from build123d import *

# Parameters (mm, degrees)
SKETCH_1_R               = 8
EXTRUDE_1_DEPTH          = 32
M6X1_0_1_D               = 5
M6X1_0_1_DEPTH           = 6
M6X1_0_1_TIP             = 1.502151548
M6X1_0_2_D               = 5
M6X1_0_2_DEPTH           = 6
M6X1_0_2_TIP             = 1.502151548
CUT_EXTRUDE_2_DEPTH      = 10
CUT_EXTRUDE_2_DEPTH_BACK = 10
SKETCH_10_W              = 1.5
SKETCH_10_H              = 35
M8X1_0_1_D               = 7


with BuildPart() as part:
    # Sketch 1 → Extrude 1 (new body)
    with BuildSketch(Plane(origin=(0, 0, 0), x_dir=(1, 0, 0), z_dir=(0, 1, 0))):
        with Locations(Location((0, 0, 0), (0, 0, 270))):
            Circle(SKETCH_1_R)
    extrude(amount=EXTRUDE_1_DEPTH)

    # M6x1.0 _1
    with Locations(Plane(origin=(0, 32, 0), x_dir=(1, 0, 0), z_dir=(0, 1, 0))):
        with Locations((0, 0)):
            Hole(M6X1_0_1_D / 2, depth=M6X1_0_1_DEPTH)
            with Locations((0, 0, -(M6X1_0_1_DEPTH + M6X1_0_1_TIP / 2))):  # 118° drill point
                Cone(0, M6X1_0_1_D / 2, M6X1_0_1_TIP, mode=Mode.SUBTRACT)

    # M6x1.0 _2
    with Locations(Plane(origin=(0, 0, 0), x_dir=(-1, 0, 0), z_dir=(0, -1, 0))):
        with Locations((0, 0)):
            Hole(M6X1_0_2_D / 2, depth=M6X1_0_2_DEPTH)
            with Locations((0, 0, -(M6X1_0_2_DEPTH + M6X1_0_2_TIP / 2))):  # 118° drill point
                Cone(0, M6X1_0_2_D / 2, M6X1_0_2_TIP, mode=Mode.SUBTRACT)

    # Sketch 10 → Cut-Extrude 2 (cut, two sides: drawn at the far end of the back side and taken through both)
    with BuildSketch(Plane.XY.offset(-CUT_EXTRUDE_2_DEPTH_BACK)):
        with Locations((7.25, 16)):
            Rectangle(SKETCH_10_W, SKETCH_10_H)
        with Locations((-7.25, 16)):
            Rectangle(SKETCH_10_W, SKETCH_10_H)
    extrude(amount=CUT_EXTRUDE_2_DEPTH + CUT_EXTRUDE_2_DEPTH_BACK, mode=Mode.SUBTRACT)

    # M8x1.0 _1 (through all)
    with Locations(Plane(origin=(6.5, 0, 0), x_dir=(0, 0, -1), z_dir=(1, 0, 0))):
        with Locations((0, 16)):
            Hole(M8X1_0_1_D / 2)


solid = part.part
Here's how the part is built. I have some questions about the finished solid (model axes, mm). A direction names the side the tool comes from. Coordinates: 2 decimals unless noted, no trailing zeros. Order: outer loops, then holes, each group sorted by start corner. A loop starts at its lowest first (then second) coordinate and runs counter-clockwise, first axis right, second up. Notation, with made-up numbers: M 45,17 L 99,17 A17 ccw 99,32 Z; hole C 8.25,-29 d3. An arc over 180 degrees is marked long. Answer as CSV lines item,"result".
Item 1: On a 3-axis mill with a long thin cutter (end or side, diameter ignored), from which of +Z, -Z, +X, -X, +Y, -Y can I reach the whole of each face in a straight line? I mean faces 5 (the face through (0.54, 28.96, 2.44)), 6 (the face through (-0.54, 3.04, 2.44)), 7 (the face through (-0.09, 19.47, -0.46)). Say none if no direction works.
Results found:
face 5,"+Y"
face 6,"-Y"
face 7,"+X, -X"
Item 2: We'd pull the mould along X, two halves only. Please class faces 1 (the face through (0.094, 7.241, 0.424)), 2 (the face through (0, 16, 8)), 3 (the face through (-3, 0, 0)), 4 (the face through (-6.5, 12, 0)): +X half, -X half, draft (parallel to the pull), parting line (faces both ways), or undercut.
Results found:
face 1,"undercut"
face 2,"parting line"
face 3,"draft"
face 4,"-X half"
Item 3: For pin 1 (6 mm diameter, centred on x = 2.5, y = 4.5, fed in from -Z); pin 2 (3 mm diameter, centred on x = -3.5, y = 9.5, fed in from -Z); pin 3 (3 mm diameter, centred on x = 0, z = 0, fed in from -Y); pin 4 (1 mm diameter, centred on x = -1.5, y = 25, fed in from +Z), each with a flat end and sliding along its axis, tell me the tip position at first contact or that it passes through.
Results found:
pin 1,"z = -8"
pin 2,"z = -7.75"
pin 3,"y = 6.6"
pin 4,"z = 7.94"
Item 4: Imagine slicing it at B-B on y = 16. Write out the boundary of the cut face in (x, z).
Results found:
outline,"M -6.5,-4.66 A8 ccw 6.5,-4.66 L 6.5,-3.5 L -6.5,-3.5 Z; M -6.5,3.5 L 6.5,3.5 L 6.5,4.66 A8 ccw -6.5,4.66 Z"
Item 5: If I drill on line 1 (Z direction, x = 0, y = 2.85); line 2 (Z direction, x = 0.25, y = 22.5); line 3 (Y direction, x = 3.25, z = -1), over which ranges is the centre line in solid material (lowest first)?
Results found:
line 1,"-8 to -2.5, 2.5 to 8"
line 2,"-8 to 8"
line 3,"0 to 12.65, 19.35 to 32"
Item 6: Imagine slicing it at C-C on y = 9.5. Write out the boundary of the cut face in (x, z).
Results found:
outline,"M -6.5,-4.66 A8 ccw 6.5,-4.66 L 6.5,4.66 A8 ccw -6.5,4.66 Z"
Item 7: Imagine slicing it at A-A on y = 29.5. Write out the boundary of the cut face in (x, z).
Results found:
outline,"M -6.5,-4.66 A8 ccw 6.5,-4.66 L 6.5,4.66 A8 ccw -6.5,4.66 Z; hole C 0,0 d5"
Item 8: Imagine slicing it at D-D on z = 5. Write out the boundary of the cut face in (x, y) (3 decimals), plus the area to 3 significant figures.
Results found:
outline,"M -6.245,0 L 6.245,0 L 6.245,32 L -6.245,32 Z"
area,"400 mm2"
